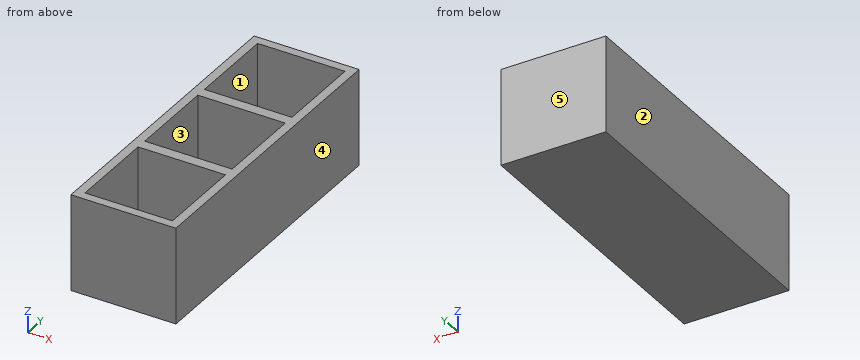
from build123d import *

# Parameters (mm, degrees)
CROQUIS1_W              = 48
CROQUIS1_H              = 138
SALIENTE_EXTRUIR1_DEPTH = 44
VACIADO1_T              = -4
CROQUIS2_W              = 40
CROQUIS2_H              = 5
SALIENTE_EXTRUIR2_DEPTH = 40


with BuildPart() as part:
    # Croquis1 → Saliente-Extruir1 (new body)
    with BuildSketch(Plane.XY):
        with Locations((24, 69)):
            Rectangle(CROQUIS1_W, CROQUIS1_H)
    extrude(amount=SALIENTE_EXTRUIR1_DEPTH)

    # Vaciado1
    vaciado1_openings = [part.faces().sort_by_distance(p)[0] for p in [
        (24, 69, 44),
    ]]
    offset(amount=VACIADO1_T, openings=vaciado1_openings, kind=Kind.INTERSECTION)

    # Croquis2 → Saliente-Extruir2 (add, through all)
    with BuildSketch(Plane.XY.offset(4)):
        with Locations((24, 46.5)):
            Rectangle(CROQUIS2_W, CROQUIS2_H)
        with Locations((24, 91.5)):
            Rectangle(CROQUIS2_W, CROQUIS2_H)
    extrude(amount=SALIENTE_EXTRUIR2_DEPTH)


solid = part.part
Read the model definition and answer for the solid it produces. Units are mm, in the model's axes. Face numbers are marked on the shaded views. A direction names the side the tool comes from. Give positions to 0.01 mm unless a question says otherwise; leave off trailing zeros. Write each loop counter-clockwise with the first axis right and the second up, starting at its lowest first coordinate (ties: lowest second). Pieces come first, ordered by that corner, then holes. Notation, with made-up numbers: (9.5, 50) - (38.5, 50) arc R35 ccw to (38.5, 86) - close; hole circle Ø8 at (-25, 55). An arc over 180 degrees is marked (long way). Answer in a Markdown table with one row per item. Add a question column.
Item 1: Determine the mould class of the marked faces 3, 4 and 5 for opening direction X: pulls with the +X half, pulls with the -X half, needs draft (parallel to the pull), parting line crosses it, or undercut.
Item 2: A flat-ended cylindrical pin translates along its axis: P1, Ø6, axis at x = 33.5, y = 82, coming from the +Z side. Find the tip coordinate at first contact, or state that the pin passes through.
Item 3: Section B-B, the plane y = 51.5 is taken. Write down the section's boundary in (x, z), and give its area (3 significant figures).
Item 4: A tool of negligible diameter and unlimited length cuts with its end or side. For the marked faces 1 and 2, from which of +Z, -Z, +X, -X, +Y, -Y can it reach the whole face along a straight path? Write none if from no direction.
Item 5: Section C-C, the plane x = 28 is taken. Write down the section's boundary in (y, z).
Item 6: Find the intervals of material crossed by L1, parallel to Y at x = 37, z = 17.5; L2, parallel to X at y = 20, z = 14.5; L3, parallel to Z at x = 17.5, y = 42, in increasing order.
Item 7: Section A-A, the plane z = 16 is taken. Write down the section's boundary in (x, y).
Recorded:
| question | item | result |
|---|---|---|
| 1 | face 3 | undercut |
| 1 | face 4 | pulls with the +X half |
| 1 | face 5 | needs draft |
| 2 | P1 | stops at z = 4 |
| 3 | outline | (0, 0) - (48, 0) - (48, 44) - (44, 44) - (44, 4) - (4, 4) - (4, 44) - (0, 44) - close |
| 3 | area | 512 mm2 |
| 4 | face 1 | +Z |
| 4 | face 2 | +Z, -Z, -X, +Y, -Y |
| 5 | outline | (0, 0) - (138, 0) - (138, 44) - (134, 44) - (134, 4) - (94, 4) - (94, 44) - (89, 44) - (89, 4) - (49, 4) - (49, 44) - (44, 44) - (44, 4) - (4, 4) - (4, 44) - (0, 44) - close |
| 6 | L1 | y = 0 to 4, 44 to 49, 89 to 94, 134 to 138 |
| 6 | L2 | x = 0 to 4, 44 to 48 |
| 6 | L3 | z = 0 to 4 |
| 7 | outline | (0, 0) - (48, 0) - (48, 138) - (0, 138) - close; hole (4, 4) - (44, 4) - (44, 44) - (4, 44) - close; hole (4, 49) - (44, 49) - (44, 89) - (4, 89) - close; hole (4, 94) - (44, 94) - (44, 134) - (4, 134) - close |
